The model under review builds one solid part; all positions refer to its coordinate system, in mm. A direction names the side the tool comes from. Coordinates: 2 decimals unless noted, no trailing zeros. Order: outer loops, then holes, each group sorted by start corner. A loop starts at its lowest first (then second) coordinate and runs counter-clockwise, first axis right, second up. Notation, with made-up numbers: (56, 50) -> (115, 50) arc R18 ccw to (115, 80) -> close; hole circle Ø6 at (17, 76.5). An arc over 180 degrees is marked (long way). Put each result on its own line as item: value.
from build123d import *

# Parameters (mm, degrees)
SKETCH_3_W              = 20
SKETCH_3_H              = 20
SKETCH_3_W_2            = 16.4
SKETCH_3_H_2            = 16.4
EXTRUDE_1_DEPTH         = 120
HOLE_WIZARD_4_2_4_2_1_D = 4.2
CUT_EXTRUDE_START       = -20
CUT_EXTRUDE_1_DEPTH     = 20
CUT_EXTRUDE_2_REACH     = 125.288
SKETCH_8_R              = 6


# Read off the part's stored shape, not the designer's step: 切除-拉伸1
with BuildPart() as part:
    # 草图3 → 凸台-拉伸1 (new body)
    with BuildSketch(Plane.XY):
        with Locations((10, 10)):
            Rectangle(SKETCH_3_W, SKETCH_3_H)
        with Locations((10, 10)):
            Rectangle(SKETCH_3_W_2, SKETCH_3_H_2, mode=Mode.SUBTRACT)
    extrude(amount=-EXTRUDE_1_DEPTH)

    # Ø4.2 (4.2) 直径孔1 (through all)
    with Locations(Plane(origin=(10, 0, -105), x_dir=(0, 0, -1), z_dir=(0, -1, 0))):
        with Locations((0, 0), (-35, 0), (-55, 0), (-90, 0)):
            Hole(HOLE_WIZARD_4_2_4_2_1_D / 2)

    # 切除-拉伸1 outline → 切除-拉伸1 (cut)
    with BuildSketch(Plane(origin=(20, 0, 0), x_dir=(0, 0, -1), z_dir=(1, 0, 0)).offset(CUT_EXTRUDE_START)):
        with BuildLine():
            ThreePointArc((45, 17), (38, 10), (45, 3))
            Line((45, 3), (75, 3))
            ThreePointArc((75, 3), (82, 10), (75, 17))
            Line((75, 17), (45, 17))
        make_face()
    extrude(amount=CUT_EXTRUDE_1_DEPTH, mode=Mode.SUBTRACT)

    # 草图8 → 切除-拉伸2 (cut, up to next)
    with BuildSketch(Plane.XZ.offset(-20), mode=Mode.PRIVATE) as cut_extrude_2_sk1:
        with Locations(Location((10, -105, 0), (0, 0, 90))):
            Circle(SKETCH_8_R)
    cut_extrude_2_tool1 = extrude(cut_extrude_2_sk1.sketch, amount=CUT_EXTRUDE_2_REACH, mode=Mode.PRIVATE) & part.part
    # 草图8 → 切除-拉伸2 (cut, up to next)
    with BuildSketch(Plane.XZ.offset(-20), mode=Mode.PRIVATE) as cut_extrude_2_sk2:
        with Locations(Location((10, -15, 0), (0, 0, 90))):
            Circle(SKETCH_8_R)
    cut_extrude_2_tool2 = extrude(cut_extrude_2_sk2.sketch, amount=CUT_EXTRUDE_2_REACH, mode=Mode.PRIVATE) & part.part
    add(cut_extrude_2_tool1.solids().sort_by_distance((10, 20, -105))[0], mode=Mode.SUBTRACT)
    add(cut_extrude_2_tool2.solids().sort_by_distance((10, 20, -15))[0], mode=Mode.SUBTRACT)


solid = part.part
Item 1: Consider section A-A on z = -65. Write out the cut boundary in (x, y), and give its area (3 significant figures).
Answers below:
outline: (0, 0) -> (20, 0) -> (20, 3) -> (18.2, 3) -> (18.2, 1.8) -> (1.8, 1.8) -> (1.8, 3) -> (0, 3) -> close; (0, 17) -> (1.8, 17) -> (1.8, 18.2) -> (18.2, 18.2) -> (18.2, 17) -> (20, 17) -> (20, 20) -> (0, 20) -> close
area: 80.6 mm^2
Item 2: Consider section D-D on z = -8. Write out the cut boundary in (x, y).
Answers below:
outline: (0, 0) -> (20, 0) -> (20, 20) -> (0, 20) -> close; hole (1.8, 1.8) -> (18.2, 1.8) -> (18.2, 18.2) -> (1.8, 18.2) -> close
Item 3: For line 1 (X direction, y = 2.5, z = -80); line 2 (X direction, y = 19.1, z = -70), list the stretches that pass through material, from the lowest coordinate up. Write a range as from..to.
Answers below:
line 1: 0..1.8, 18.2..20
line 2: 0..7.9, 12.1..20
Item 4: For faces 1 (the cylindrical face through (10, 19, -111)), 2 (the flat face through (1, 10, -120)), 3 (the flat face through (1.8, 17.2, -59.2)), 4 (the cylindrical face through (1, 10, -38)), 5 (the cylindrical face through (12.082, 0.913, -15.273)), list the 3-axis set-ups (+Z, -Z, +X, -X, +Y, -Y) from which the entire face can be reached by the end or side of a thin tool; tool diameter is ignored.
Answers below:
face 1: +Y
face 2: -Z, +X, -X, +Y, -Y
face 3: +Z, -Z
face 4: +X, -X
face 5: +Y, -Y
Item 5: Mouldability with a two-part tool opening along Y and no side actions: class faces 6 (the flat face through (10, 18.2, -59)), 7 (the cylindrical face through (10.631, 19.113, -47.997)), 8 (the flat face through (10, 0, -59)) as +Y half, -Y half, draft (parallel to the pull), parting line (faces both ways), or undercut.
Answers below:
face 6: undercut
face 7: draft
face 8: -Y half
Item 6: Consider section B-B on x = 6. Write out the cut boundary in (y, z).
Answers below:
outline: (0, -120) -> (1.8, -120) -> (1.8, 0) -> (0, 0) -> close; (18.2, -120) -> (20, -120) -> (20, -109.47) -> (18.2, -109.47) -> close; (18.2, -100.53) -> (20, -100.53) -> (20, -19.47) -> (18.2, -19.47) -> close; (18.2, -10.53) -> (20, -10.53) -> (20, 0) -> (18.2, 0) -> close
Item 7: For pin 1 Ø4 at (x, z) = (10, -50) entering from +Y; pin 2 Ø5.5 at (x, z) = (10, -105) entering from +Y, all flat-tipped, find the tip position at first contact; note any pin that passes through.
Answers below:
pin 1: through
pin 2: y = 1.8
Item 8: Consider section C-C on y = 10. Write out the cut boundary in (x, z), and give its area (3 significant figures).
Answers below:
outline: (0, -120) -> (1.8, -120) -> (1.8, -82) -> (0, -82) -> close; (0, -38) -> (1.8, -38) -> (1.8, 0) -> (0, 0) -> close; (18.2, -120) -> (20, -120) -> (20, -82) -> (18.2, -82) -> close; (18.2, -38) -> (20, -38) -> (20, 0) -> (18.2, 0) -> close
area: 274 mm^2
